Design review of the part built by this model. Coordinates are the model's own, in mm. A direction names the side the tool comes from. Round coordinates to 2 decimals unless told otherwise and drop trailing zeros. Write each loop counter-clockwise with the first axis right and the second up, starting at its lowest first coordinate (ties: lowest second). Pieces come first, ordered by that corner, then holes. Notation, with made-up numbers: (-6, 59.25) - (45, 59.25) arc R37 cw to (45, 98.25) - close; hole circle Ø11 at (-26.75, 24). An arc over 180 degrees is marked (long way). Use one line per item in the form item = value.
```python
from build123d import *

# Parameters (mm, degrees)
F0_W     = 647.7
F0_H     = 209.55
F1_DEPTH = 50.8
F2_W     = 101.6
F2_H     = 101.6
F3_DEPTH = 25.4
F4_W     = 203.2
F4_H     = 15.24
F5_DEPTH = 116.84
F6_W     = 152.4
F6_H     = 88.9
F7_DEPTH = 152.4


with BuildPart() as f1:
    # F0 (on Front) → F1 (new body)
    with BuildSketch(Plane.XZ):
        with Locations((323.85, 104.775)):
            Rectangle(F0_W, F0_H)
    extrude(amount=F1_DEPTH)

    # F2 (on face) → F3 (join)
    with BuildSketch(Plane.XZ.offset(50.8)):
        with Locations((266.7, 158.75)):
            Rectangle(F2_W, F2_H)
    extrude(amount=F3_DEPTH)

    # F4 (on face) → F5 (join)
    with BuildSketch(Plane.XZ.offset(50.8)):
        with Locations((546.1, 68.58)):
            Rectangle(F4_W, F4_H)
    extrude(amount=F5_DEPTH)

    # F6 (on face) → F7 (join)
    with BuildSketch(Plane.XZ.offset(50.8)):
        with Locations((571.5, 165.1)):
            Rectangle(F6_W, F6_H)
    extrude(amount=F7_DEPTH)


solid = f1.part
```
Q1. For P1, Ø1.5, axis at x = 97, z = 51.5, coming from the -Y side; P2, Ø10, axis at x = 475.5, y = -71.5, coming from the -Z side; P3, Ø4.5, axis at x = 526, z = 70, coming from the -Y side, all flat-tipped, find the tip position at first contact; note any pin that passes through.
Calculated:
P1 = -50.8
P2 = 60.96
P3 = -167.64
Q2. Machinability: for faces 4 (the flat face through (495.3, -126, 164)), 5 (the flat face through (317.5, -63, 158)), 6 (the flat face through (570, -126, 120.65)), 7 (the flat face through (266, -76.2, 159)), which of the approach directions +Z, -Z, +X, -X, +Y, -Y give a long, thin tool a straight path to every point of the face, cutting with its end or side? Answer none if there is none.
Calculated:
face_4 = +Z, -Y
face_5 = +Z, -Z, -Y
face_6 = +X, -Y
face_7 = +Z, -Z, -X, -Y
Q3. We need section B-B on y = -91. Write out the cut boundary in (x, z), then the cut area to 3 significant figures.
Calculated:
outline = (444.5, 60.96) - (647.7, 60.96) - (647.7, 76.2) - (444.5, 76.2) - close; (495.3, 120.65) - (647.7, 120.65) - (647.7, 209.55) - (495.3, 209.55) - close
area = 16,600 mm2
Q4. To check wall thickness, follow line 1 along Z through (x, y) = (541.5, -61); line 2 along Y through (x, z) = (299, 200); line 3 along Y through (x, z) = (333, 106.5). State the ranges of each line that lie inside material, in increasing order. Write a range as from..to.
Calculated:
line_1 = 60.96..76.2, 120.65..209.55
line_2 = -76.2..0
line_3 = -50.8..0
Q5. We need section C-C on x = 609.5. Write out the cut boundary in (y, z), then the cut area to 3 significant figures.
Calculated:
outline = (-203.2, 120.65) - (-50.8, 120.65) - (-50.8, 76.2) - (-167.64, 76.2) - (-167.64, 60.96) - (-50.8, 60.96) - (-50.8, 0) - (0, 0) - (0, 209.55) - (-203.2, 209.55) - close
area = 26,000 mm2
Q6. Draft analysis for pull direction Z (two halves, no side actions). For faces 1 (the flat face through (545, -108, 60.96)), 2 (the flat face through (545, -167.64, 69)), 3 (the flat face through (545, -108, 76.2)), state which applies: released by +Z, released by -Z, zero draft, split by the parting line, or undercut.
Calculated:
face_1 = released by -Z
face_2 = zero draft
face_3 = undercut
Q7. We need section D-D on z = 127. Write out the cut boundary in (x, y).
Calculated:
outline = (0, -50.8) - (215.9, -50.8) - (215.9, -76.2) - (317.5, -76.2) - (317.5, -50.8) - (495.3, -50.8) - (495.3, -203.2) - (647.7, -203.2) - (647.7, 0) - (0, 0) - close
Q8. We need section A-A on y = -65. Write out the cut boundary in (x, z).
Calculated:
outline = (215.9, 107.95) - (317.5, 107.95) - (317.5, 209.55) - (215.9, 209.55) - close; (444.5, 60.96) - (647.7, 60.96) - (647.7, 76.2) - (444.5, 76.2) - close; (495.3, 120.65) - (647.7, 120.65) - (647.7, 209.55) - (495.3, 209.55) - close
